Input: dimensioned drawing with shaded views. Units: mm. Origin: part minimum x, y, z. Give positions to 0.01 mm unless a question says otherwise; leave off trailing zeros. Write each loop counter-clockwise with the first axis right and the second up, starting at its lowest first coordinate (ties: lowest second). Pieces come first, ordered by that corner, then holes.
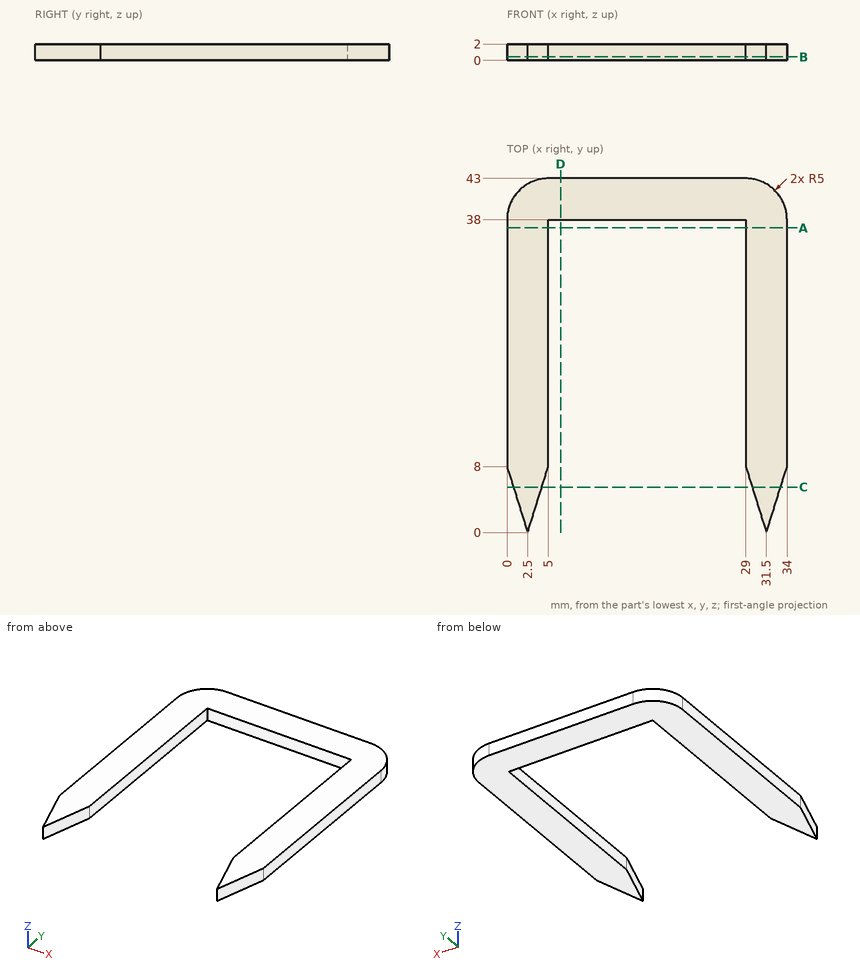
1. Line query: L1, parallel to X at y = 27, z = 0.75; L2, parallel to Y at x = 19, z = 0.25; L3, parallel to X at y = 5, z = 0.3. Output: solid intervals per line, ascending.
2. Cut plane C-C, the plane y = 5.5. Return the cut outline in (x, z).
3. Cut plane B-B, the plane z = 0.45. Return the cut outline in (x, y), then the cut area to 3 significant figures.
4. Cut plane D-D, the plane x = 6.5. Return the cut outline in (y, z).
5. Cut plane A-A, the plane y = 37. Return the cut outline in (x, z), then the cut area to 3 significant figures.
Response values:
1. L1: x = 0 to 5, 29 to 34
1. L2: y = 38 to 43
1. L3: x = 0.94 to 4.06, 29.94 to 33.06
2. outline: (0.78, 0) - (4.22, 0) - (4.22, 2) - (0.78, 2) - close; (29.78, 0) - (33.22, 0) - (33.22, 2) - (29.78, 2) - close
3. outline: (0, 8) - (2.5, 0) - (5, 8) - (5, 38) - (29, 38) - (29, 8) - (31.5, 0) - (34, 8) - (34, 38) arc R5 ccw to (29, 43) - (5, 43) arc R5 ccw to (0, 38) - close
3. area: 499 mm2
4. outline: (38, 0) - (43, 0) - (43, 2) - (38, 2) - close
5. outline: (0, 0) - (5, 0) - (5, 2) - (0, 2) - close; (29, 0) - (34, 0) - (34, 2) - (29, 2) - close
5. area: 20.0 mm2
